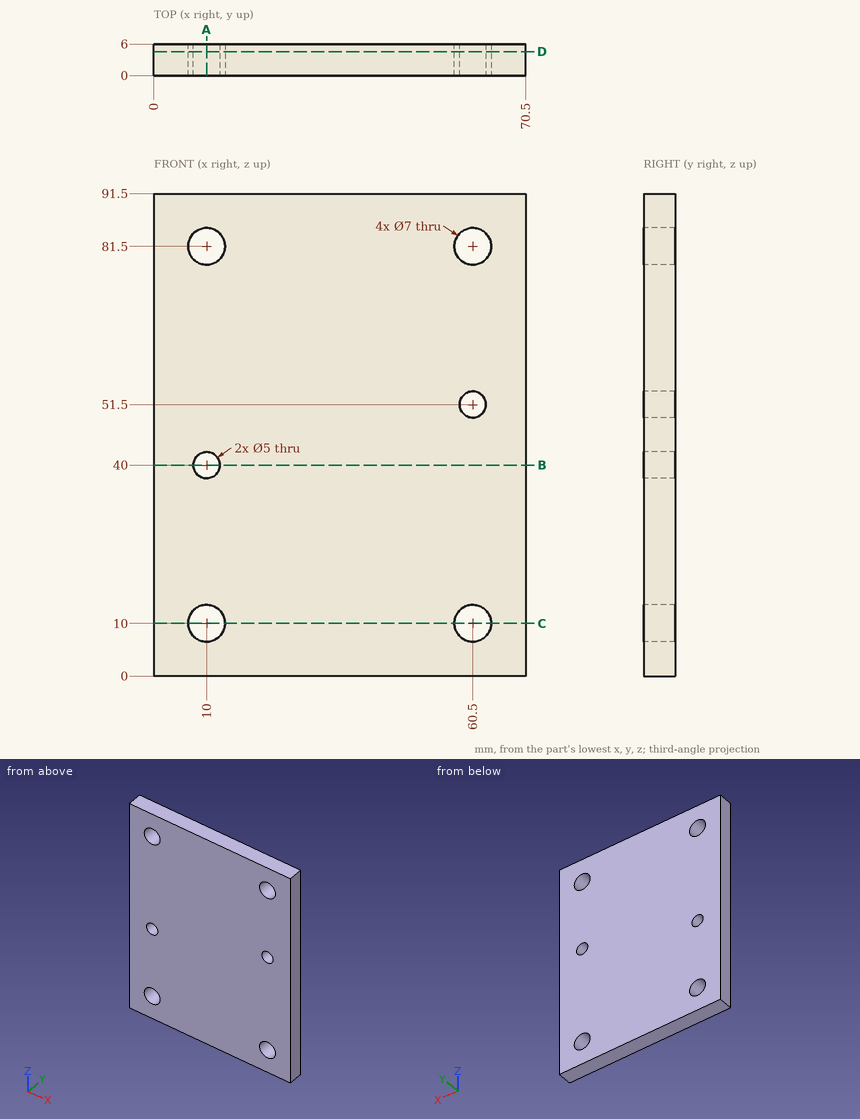
Print and shaded views of the part. All mm, measured from the part's lowest x, y and z. Give positions to 0.01 mm unless a question says otherwise; leave off trailing zeros. Loops run counter-clockwise (first coordinate to the right, second up) from the corner with the lowest first, then second, coordinate; pieces in that order, holes last.
1) Saw through at D-D (y = 4.55). Write the cut outline in (x, z).
2) Wall check: line 1 (Z direction, x = 10, y = 4.5); line 2 (Z direction, x = 60.5, y = 3.25). Give the ranges that are in metal, low to high.
3) Saw through at B-B (z = 40). Write the cut outline in (x, y), plus the area to 3 significant figures.
4) Saw through at A-A (x = 10). Write the cut outline in (y, z), plus the area to 3 significant figures.
5) Saw through at C-C (z = 10). Write the cut outline in (x, y), plus the area to 3 significant figures.
6) Flat gauge pin, fed straight in: pin 1 Ø4 at (x, z) = (60.5, 81.5) entering from +Y. Where does the tip first touch, or does it go through?
Answer block:
1. outline: (0, 0) - (70.5, 0) - (70.5, 91.5) - (0, 91.5) - close; hole circle Ø7 at (10, 10); hole circle Ø7 at (10, 81.5); hole circle Ø5 at (10, 40); hole circle Ø7 at (60.5, 10); hole circle Ø7 at (60.5, 81.5); hole circle Ø5 at (60.5, 51.5)
2. line 1: z = 0 to 6.5, 13.5 to 37.5, 42.5 to 78, 85 to 91.5
2. line 2: z = 0 to 6.5, 13.5 to 49, 54 to 78, 85 to 91.5
3. outline: (0, 0) - (7.5, 0) - (7.5, 6) - (0, 6) - close; (12.5, 0) - (70.5, 0) - (70.5, 6) - (12.5, 6) - close
3. area: 393 mm2
4. outline: (0, 0) - (6, 0) - (6, 6.5) - (0, 6.5) - close; (0, 13.5) - (6, 13.5) - (6, 37.5) - (0, 37.5) - close; (0, 42.5) - (6, 42.5) - (6, 78) - (0, 78) - close; (0, 85) - (6, 85) - (6, 91.5) - (0, 91.5) - close
4. area: 435 mm2
5. outline: (0, 0) - (6.5, 0) - (6.5, 6) - (0, 6) - close; (13.5, 0) - (57, 0) - (57, 6) - (13.5, 6) - close; (64, 0) - (70.5, 0) - (70.5, 6) - (64, 6) - close
5. area: 339 mm2
6. pin 1: passes through
